from build123d import *

# Parameters (mm, degrees)
SKETCH016_R       = 1.85
EXTRUDE013_DEPTH  = 12
CYLINDER007_R     = 5
CYLINDER007_DEPTH = 1
EXTRUDE012_DEPTH  = 15


with BuildPart() as extrude013:
    # Sketch016 → Extrude013 (new body)
    with BuildSketch(Plane.XZ):
        Polygon((11.75, 36), (11.75, 19), (-17.25, 19), (-23.25, 25), (-23.25, 30), (-17.25, 36), align=None)
        with Locations((-16, 27.481564)):
            Circle(SKETCH016_R, mode=Mode.SUBTRACT)
    extrude(amount=-EXTRUDE013_DEPTH)


with BuildPart() as unprintable:
    # Cylinder007 → Cylinder007 (new body)
    with BuildSketch(Plane(origin=(-16, 18, 27.5), x_dir=(1, 0, 0), z_dir=(0, -1, 0))):
        Circle(CYLINDER007_R)
    extrude(amount=CYLINDER007_DEPTH)


with BuildPart() as body007:
    # Sketch015 → Extrude012 (new body)
    with BuildSketch(Plane.XY.offset(50)):
        with BuildLine():
            ThreePointArc((8.75, 0), (1.006685, 8.691898), (-8.518363, 2))
            Line((-8.518363, 2), (-22.518363, 2))
            Line((-22.518363, 4.5), (-22.518363, 2))
            Line((-10.310795, 4.5), (-22.518363, 4.5))
            ThreePointArc((11.25, 0), (2.298483, 11.012696), (-10.310795, 4.5))
            Line((8.75, 0), (11.25, 0))
        make_face()
    extrude(amount=EXTRUDE012_DEPTH)


with BuildPart() as body007_1:
    # Extrude012 placement: moved
    add(body007.part.moved(Location((0, 0, -30))))

    # Fusion016: union unprintable
    add(unprintable.part)

    # Common001: intersect Extrude013
    add(extrude013.part, mode=Mode.INTERSECT)


with BuildPart() as part_mirroring008:
    # Part__Mirroring008: instance of Body007
    add(body007_1.part.mirror(Plane(origin=(0, 0, 0), x_dir=(1, 0, 0), z_dir=(0, 1, 0))))


solid = part_mirroring008.part
For this review, take the finished solid that the model builds, in its own axes (mm). A direction names the side the tool comes from. Coordinates: 2 decimals unless noted, no trailing zeros. Order: outer loops, then holes, each group sorted by start corner. A loop starts at its lowest first (then second) coordinate and runs counter-clockwise, first axis right, second up. Notation, with made-up numbers: (54, 4.5) - (108, 4.5) arc R27 cw to (108, 31.5) - close; hole circle Ø4 at (6.25, -31). An arc over 180 degrees is marked (long way). Use one line per item in the form item = value.
Q1. Consider section B-B (y = -2.5). Give the boundary of the cut face in (x, z).
Checked values:
outline = (-22.52, 24.27) - (-18.25, 20) - (-8.39, 20) - (-8.39, 35) - (-18.25, 35) - (-22.52, 30.73) - close; (8.39, 20) - (10.97, 20) - (10.97, 35) - (8.39, 35) - close; hole circle Ø3.7 at (-16, 27.48)
Q2. Consider section D-D (z = 31.25). Give the boundary of the cut face in (x, y), then the cut area to 3 significant figures.
Checked values:
outline = (-22, -4.5) - (-10.31, -4.5) arc R11.25 ccw to (11.25, 0) - (8.75, 0) arc R8.75 cw to (-8.52, -2) - (-22, -2) - close
area = 102 mm2
Q3. For probe 1 along Z at (x, y) = (-16, -2.9); probe 2 along Y at (x, z) = (-14.5, 31); probe 3 along X at (y, z) = (-5, 33), list the stretches that pass through material, from the lowest coordinate up. Write a range as from..to.
Checked values:
probe_1 = 20..25.63, 29.33..35
probe_2 = -4.5..-2
probe_3 = -10.08..-7.18, 7.18..10.08
Q4. Consider section A-A (x = -16). Give the boundary of the cut face in (y, z), then the cut area to 4 significant figures.
Checked values:
outline = (-4.5, 20) - (-2, 20) - (-2, 25.63) - (-4.5, 25.63) - close; (-4.5, 29.33) - (-2, 29.33) - (-2, 35) - (-4.5, 35) - close
area = 28.25 mm2
Q5. Consider section C-C (y = -6.25). Give the boundary of the cut face in (x, z), then the cut area to 3 significant figures.
Checked values:
outline = (-9.35, 20) - (-6.12, 20) - (-6.12, 35) - (-9.35, 35) - close; (6.12, 20) - (9.35, 20) - (9.35, 35) - (6.12, 35) - close
area = 96.9 mm2
Q6. For P1, Ø6, axis at x = -14, z = 22, coming from the +Y side; P2, Ø3, axis at x = 2, z = 31, coming from the -Y side; P3, Ø1, axis at y = -9, z = 22.5, coming from the +X side, all flat-tipped, find the tip position at first contact; note any pin that passes through.
Checked values:
P1 = -2
P2 = -11.24
P3 = 7.37
Q7. For faces 1 (the flat face through (-14, -2, 27)), 2 (the flat face through (-3, -9, 20)), list the 3-axis set-ups (+Z, -Z, +X, -X, +Y, -Y) from which the entire face can be reached by the end or side of a thin tool; tool diameter is ignored.
Checked values:
face_1 = +Z, -Z, -X, +Y
face_2 = -Z, +X, -X, +Y, -Y
Q8. Draft analysis for pull direction Z (two halves, no side actions). For faces 3 (the flat face through (-20.35, -3.23, 22.1)), 4 (the flat face through (-3, -9, 35)), 5 (the flat face through (-15, -4.5, 25.7)), 6 (the cylindrical face through (-15.15, -3.23, 25.84)), state which applies: +Z half, -Z half, draft (parallel to the pull), parting line (faces both ways), or undercut.
Checked values:
face_3 = -Z half
face_4 = +Z half
face_5 = draft
face_6 = undercut
